Verification items for this drawing (mm, ordinates from the low corner). Give positions to 0.01 mm unless a question says otherwise; leave off trailing zeros. Write each loop counter-clockwise with the first axis right and the second up, starting at its lowest first coordinate (ties: lowest second). Pieces come first, ordered by that corner, then holes. Notation, with made-up numbers: (41.25, -1) -> (46.25, -1) arc R6 cw to (46.25, 7) -> close; hole circle Ø3 at (-26, 19). An arc over 180 degrees is marked (long way). Answer as a JSON object with one key per item and string values.
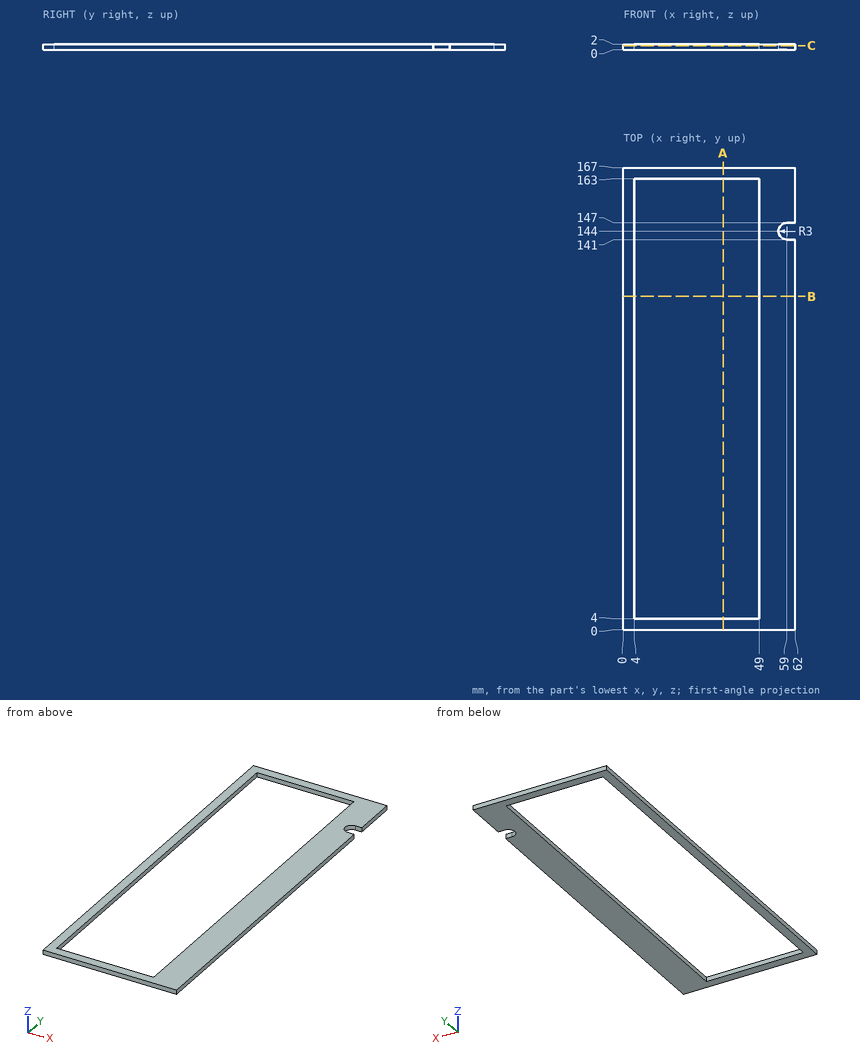
1. Sectioned sample at B-B, the plane y = 120.5. Enter the section's corners in (x, z), plus the area to 3 significant figures.
Determined:
{"outline": "(0, 0) -> (4, 0) -> (4, 2) -> (0, 2) -> close; (49, 0) -> (62, 0) -> (62, 2) -> (49, 2) -> close", "area": "34.0 mm^2"}
2. Sectioned sample at C-C, the plane z = 1.4. Enter the section's corners in (x, y), plus the area to 3 significant figures.
Determined:
{"outline": "(0, 0) -> (62, 0) -> (62, 141) -> (59, 141) arc R3 cw to (59, 147) -> (62, 147) -> (62, 167) -> (0, 167) -> close; hole (4, 4) -> (49, 4) -> (49, 163) -> (4, 163) -> close", "area": "3,170 mm^2"}
3. Sectioned sample at A-A, the plane x = 36. Enter the section's corners in (y, z), plus the area to 3 significant figures.
Determined:
{"outline": "(0, 0) -> (4, 0) -> (4, 2) -> (0, 2) -> close; (163, 0) -> (167, 0) -> (167, 2) -> (163, 2) -> close", "area": "16.0 mm^2"}
4. Scan lines: L1, parallel to X at y = 74.5, z = 1.3; L2, parallel to Y at x = 19, z = 1.85. Record each from-to range of solid material in increasing order. Write a range as [from, to].
Determined:
{"L1": "[0, 4], [49, 62]", "L2": "[0, 4], [163, 167]"}
